Check sheet for the modelled part. Datum: model origin and axes. Units: mm. A direction names the side the tool comes from. Coordinates: 2 decimals unless noted, no trailing zeros. Write each loop counter-clockwise with the first axis right and the second up, starting at its lowest first coordinate (ties: lowest second). Pieces come first, ordered by that corner, then holes. Notation, with made-up numbers: M 28.5,40.5 L 62.5,40.5 A12 ccw 62.5,46.5 Z; hole C 61.5,-12 d8. An arc over 180 degrees is marked long. Answer as CSV lines item,"result". Start each with the question number.
1) Section check B-B (y = 7). Record the cut outline in (x, z).
2) Section check C-C (y = 1.75). Record the cut outline in (x, z), and give its area (3 significant figures).
3) Access from +Z, -Z, +X, -X, +Y, -Y to the whole of each face (thin tool, end or side, straight path). Record for faces 4 (the flat face through (-0.9, 2.7, -5)), 5 (the cylindrical face through (-50, 6, 0)), 6 (the flat face through (33, 2, 2.2)).
4) Go/stop test with a flat-tipped pin: pin 1 Ø3 at (x, z) = (-40.5, 2.5) entering from +Y. Record where the tip stops, or that it passes through.
5) Section check A-A (x = -30.5). Record the cut outline in (y, z).
6) Draft check along X on faces 1 (the flat face through (-60, 5, -2.2)), 2 (the cylindrical face through (-70, 5, 0)), 3 (the cylindrical face through (70, 5, 0)). Enter one of: +X half, -X half, draft (parallel to the pull), parting line (faces both ways), or undercut.
7) Material ranges on L1, parallel to Z at x = -61, y = 5; L2, parallel to X at y = 5.5, z = 1.5; L3, parallel to X at y = 8.5, z = -4.25, recorded low to high. Write a range as [from, to].
8) Section check D-D (z = 3.5). Record the cut outline in (x, y), and give its area (3 significant figures).
from build123d import *

# Parameters (mm, degrees)
EXTRUDE_1_DEPTH     = 3
EXTRUDE_2_DEPTH     = 7
CUT_EXTRUDE_1_DEPTH = 71.887234394
CUT_EXTRUDE_2_DEPTH = 71.52659073


with BuildPart() as part:
    # 草图1 → 凸台-拉伸1 (new body)
    with BuildSketch(Plane(origin=(0, 0, 0), x_dir=(1, 0, 0), z_dir=(0, 1, 0))):
        with BuildLine():
            Line((-65, 5), (65, 5))
            ThreePointArc((65, 5), (70, 0), (65, -5))
            Line((65, -5), (-65, -5))
            ThreePointArc((-65, -5), (-70, 0), (-65, 5))
        make_face()
    extrude(amount=EXTRUDE_1_DEPTH)

    # 草图2 → 凸台-拉伸2 (add)
    with BuildSketch(Plane(origin=(0, 3, 0), x_dir=(1, 0, 0), z_dir=(0, 1, 0))):
        with BuildLine():
            Line((-65, 5), (-55, 5))
            ThreePointArc((-55, 5), (-50, 0), (-55, -5))
            Line((-55, -5), (-65, -5))
            ThreePointArc((-65, -5), (-70, 0), (-65, 5))
        make_face()
        with BuildLine():
            Line((65, 5), (55, 5))
            ThreePointArc((55, 5), (50, 0), (55, -5))
            Line((55, -5), (65, -5))
            ThreePointArc((65, -5), (70, 0), (65, 5))
        make_face()
    extrude(amount=EXTRUDE_2_DEPTH)

    # 草图3 → 切除-拉伸1 (cut, through all)
    with BuildSketch(Plane(origin=(0, 10, 0), x_dir=(1, 0, 0), z_dir=(0, 1, 0))):
        with BuildLine():
            Line((-65, 2.2), (-55, 2.2))
            ThreePointArc((-55, 2.2), (-52.8, 0), (-55, -2.2))
            Line((-55, -2.2), (-65, -2.2))
            ThreePointArc((-65, -2.2), (-67.2, 0), (-65, 2.2))
        make_face()
        with BuildLine():
            Line((65, 2.2), (55, 2.2))
            ThreePointArc((55, 2.2), (52.8, 0), (55, -2.2))
            Line((55, -2.2), (65, -2.2))
            ThreePointArc((65, -2.2), (67.2, 0), (65, 2.2))
        make_face()
    extrude(amount=-CUT_EXTRUDE_1_DEPTH, mode=Mode.SUBTRACT)

    # 草图4 → 切除-拉伸2 (cut, through all)
    with BuildSketch(Plane(origin=(0, 3, 0), x_dir=(1, 0, 0), z_dir=(0, 1, 0))):
        with BuildLine():
            Line((-41, 2.2), (-25, 2.2))
            ThreePointArc((-25, 2.2), (-22.8, 0), (-25, -2.2))
            Line((-25, -2.2), (-41, -2.2))
            ThreePointArc((-41, -2.2), (-43.2, 0), (-41, 2.2))
        make_face()
        with BuildLine():
            Line((41, 2.2), (25, 2.2))
            ThreePointArc((25, 2.2), (22.8, 0), (25, -2.2))
            Line((25, -2.2), (41, -2.2))
            ThreePointArc((41, -2.2), (43.2, 0), (41, 2.2))
        make_face()
    extrude(amount=-CUT_EXTRUDE_2_DEPTH, mode=Mode.SUBTRACT)


solid = part.part
Results found:
1,outline,"M -65,-5 L -55,-5 A5 ccw -55,5 L -65,5 A5 ccw Z; M 55,-5 L 65,-5 A5 ccw 65,5 L 55,5 A5 ccw Z; hole M -65,-2.2 L -55,-2.2 A2.2 ccw -55,2.2 L -65,2.2 A2.2 ccw Z; hole M 55,-2.2 L 65,-2.2 A2.2 ccw 65,2.2 L 55,2.2 A2.2 ccw Z"
2,outline,"M -65,-5 L 65,-5 A5 ccw 65,5 L -65,5 A5 ccw Z; hole M -65,-2.2 L -55,-2.2 A2.2 ccw -55,2.2 L -65,2.2 A2.2 ccw Z; hole M -41,-2.2 L -25,-2.2 A2.2 ccw -25,2.2 L -41,2.2 A2.2 ccw Z; hole M 25,-2.2 L 41,-2.2 A2.2 ccw 41,2.2 L 25,2.2 A2.2 ccw Z; hole M 55,-2.2 L 65,-2.2 A2.2 ccw 65,2.2 L 55,2.2 A2.2 ccw Z"
2,area,"1,090 mm2"
3,face 4,"-Z, +X, -X, +Y, -Y"
3,face 5,"+Y"
3,face 6,"+Y, -Y"
4,pin 1,"stops at y = 3"
5,outline,"M 0,-5 L 3,-5 L 3,-2.2 L 0,-2.2 Z; M 0,2.2 L 3,2.2 L 3,5 L 0,5 Z"
6,face 1,"undercut"
6,face 2,"-X half"
6,face 3,"+X half"
7,L1,"z = [-5, -2.2], [2.2, 5]"
7,L2,"x = [-69.77, -66.61], [-53.39, -50.23], [50.23, 53.39], [66.61, 69.77]"
7,L3,"x = [-67.63, -52.37], [52.37, 67.63]"
8,outline,"M -68.57,0 L 68.57,0 L 68.57,10 L 51.43,10 L 51.43,3 L -51.43,3 L -51.43,10 L -68.57,10 Z"
8,area,"651 mm2"
